from build123d import *

# Parameters (mm, degrees)
SKETCH1_R           = 7.5
BOSS_EXTRUDE1_DEPTH = 20
SKETCH2_W           = 20
SKETCH2_H           = 15
BOSS_EXTRUDE2_DEPTH = 25.5
SKETCH3_R           = 5.5
CUT_EXTRUDE1_DEPTH  = 26
SKETCH4_R           = 1.5
CUT_EXTRUDE2_DEPTH  = 30
SKETCH5_R           = 1.5
CUT_EXTRUDE3_DEPTH  = 30


with BuildPart() as part:
    # Sketch1 → Boss-Extrude1 (new body)
    with BuildSketch(Plane.XY):
        Circle(SKETCH1_R)
    extrude(amount=BOSS_EXTRUDE1_DEPTH)

    # Sketch2 → Boss-Extrude2 (add)
    with BuildSketch(Plane(origin=(0, 0, 0), x_dir=(0, 0, -1), z_dir=(1, 0, 0))):
        with Locations((-10, 0)):
            Rectangle(SKETCH2_W, SKETCH2_H)
    extrude(amount=BOSS_EXTRUDE2_DEPTH)

    # Sketch3 → Cut-Extrude1 (cut)
    with BuildSketch(Plane.XY.offset(20)):
        Circle(SKETCH3_R)
    extrude(amount=-CUT_EXTRUDE1_DEPTH, mode=Mode.SUBTRACT)

    # Sketch4 → Cut-Extrude2 (cut)
    with BuildSketch(Plane(origin=(0, 7.5, 0), x_dir=(1, 0, 0), z_dir=(0, 1, 0))):
        with Locations(Location((20.5, -10, 0), (0, 0, 270))):
            Circle(SKETCH4_R)
    extrude(amount=-CUT_EXTRUDE2_DEPTH, mode=Mode.SUBTRACT)

    # Sketch5 → Cut-Extrude3 (cut)
    with BuildSketch(Plane(origin=(0, 0, 0), x_dir=(-1, 0, 0), z_dir=(0, 0, -1))):
        with Locations((-20.5, 0)):
            Circle(SKETCH5_R)
    extrude(amount=-CUT_EXTRUDE3_DEPTH, mode=Mode.SUBTRACT)


solid = part.part
Design review of the part built by this model. Coordinates are the model's own, in mm. Give positions to 0.01 mm unless a question says otherwise; leave off trailing zeros. Order: outer loops, then holes, each group sorted by start corner. A loop starts at its lowest first (then second) coordinate and runs counter-clockwise, first axis right, second up.
1. Add section B-B, the plane x = 20.5. State the section outline as (y, z) points, then the cut area to 3 significant figures.
Solution:
outline: (-7.5, 0) - (-1.5, 0) - (-1.5, 8.5) - (-7.5, 8.5) - close; (-7.5, 11.5) - (-1.5, 11.5) - (-1.5, 20) - (-7.5, 20) - close; (1.5, 0) - (7.5, 0) - (7.5, 8.5) - (1.5, 8.5) - close; (1.5, 11.5) - (7.5, 11.5) - (7.5, 20) - (1.5, 20) - close
area: 204 mm2
2. Add section D-D, the plane y = -6. State the section outline as (x, z) points.
Solution:
outline: (-4.5, 0) - (25.5, 0) - (25.5, 20) - (-4.5, 20) - close; hole circle Ø3 at (20.5, 10)
3. Add section A-A, the plane y = 4.5. State the section outline as (x, z) points.
Solution:
outline: (-6, 0) - (-3.16, 0) - (-3.16, 20) - (-6, 20) - close; (3.16, 0) - (25.5, 0) - (25.5, 20) - (3.16, 20) - close; hole circle Ø3 at (20.5, 10)
4. To check wall thickness, follow L1, parallel to Y at x = 0, z = 7.5; L2, parallel to Z at x = 20.5, y = 5.75; L3, parallel to Y at x = 20.5, z = 4. State the ranges of each line that lie inside material, in increasing order.
Solution:
L1: y = -7.5 to -5.5, 5.5 to 7.5
L2: z = 0 to 8.5, 11.5 to 20
L3: y = -7.5 to -1.5, 1.5 to 7.5
5. Add section C-C, the plane z = 15. State the section outline as (x, y) points, then the cut area to 3 significant figures.
Solution:
outline: (0, -7.5) - (25.5, -7.5) - (25.5, 7.5) - (0, 7.5) arc R7.5 ccw to start; hole circle Ø11 at (0, 0); hole circle Ø3 at (20.5, 0)
area: 369 mm2
6. For pin 1 Ø8 at (y, z) = (1.5, 3.5) entering from -X, flat-tipped, find the tip position at first contact; note if it passes through.
Solution:
pin 1: stops at x = -7.5
7. Mouldability with a two-part tool opening along X and no side actions: class faces 1 (the cylindrical face through (-7.5, 0.16, 9.86)), 2 (the flat face through (12, 0, 20)), 3 (the cylindrical face through (20.57, -4.53, 8.5)) as +X half, -X half, draft (parallel to the pull), parting line (faces both ways), or undercut.
Solution:
face 1: -X half
face 2: draft
face 3: undercut
